Autodesk Inventor part; units mm, degrees
ref_plane "Work Plane1" through (0, 50, 0) normal (0, 1, 0) x (1, 0, 0)
ref_plane "YZ Plane" through (0, 0, 0) normal (1, 0, 0) x (0, 1, 0)
ref_plane "XZ Plane" through (0, 0, 0) normal (0, 1, 0) x (-1, 0, 0)
sketch "Sketch1" plane through (0, 0, 0) normal (0, 1, 0) x (-1, 0, 0)
  circle A0 centre (0, 0) radius 46
  dimension "d0" = 92
extrude "Extrusion1" add sketch "Sketch1" along normal blind 50
ref_plane "Work Plane1" through (0, 50, 0) normal (0, 1, 0) x (1, 0, 0)
sketch "Sketch2" plane through (0, 50, 0) normal (0, 1, 0) x (1, 0, 0)
  circle A0 centre (0, 0) radius 36
  dimension "d4" = 72
extrude "Extrusion2" cut sketch "Sketch2" against normal blind 40
sketch "Sketch3" plane through (0, 0, 0) normal (1, 0, 0) x (0, 1, 0)
  line L0 (50, -46) -> (0, -46)
  line L1 (0, -46) -> (0, 46)
  line L2 (0, 46) -> (50, 46)
  line L3 (50, 46) -> (50, 36)
  line L4 (50, 36) -> (10, 36)
  line L5 (10, 36) -> (10, -36)
  line L6 (10, -36) -> (50, -36)
  line L7 (50, -36) -> (50, -46)
  line L8 (0, 46) -> (50, 46)
  line L9 (10, 46) -> (5, 46)
  line L10 (5, 46) -> (5, 44)
  line L11 (5, 44) -> (10, 44)
  line L12 (10, 44) -> (10, 46)
  line L13 (20, 46) -> (15, 46)
  line L14 (15, 46) -> (15, 44)
  line L15 (15, 44) -> (20, 44)
  line L16 (20, 44) -> (20, 46)
  line L17 (-10, 0) -> (60, 0)
  point P0 (0, 0)
  point P1 (15, 46)
  dimension "d7" = 5
  dimension "d8" = 5
  dimension "d9" = 5
  dimension "d10" = 5
  dimension "d11" = 2
revolve "Revolution1" cut sketch "Sketch3" angle 360 about axis through (0, -10, 0) along (0, 1, 0) contours L2 L12 L11 L10 | L2 L16 L15 L14
sketch "Sketch4" plane through (0, 0, 0) normal (1, 0, 0) x (0, 1, 0)
  line L0 (10, -36) -> (50, -36)
  line L1 (50, -36) -> (50, -46)
  line L2 (50, -46) -> (20, -46)
  line L3 (20, -46) -> (20, -44)
  line L4 (20, -44) -> (15, -44)
  line L5 (15, -44) -> (15, -46)
  line L6 (15, -46) -> (10, -46)
  line L7 (10, -46) -> (10, -44)
  line L8 (10, -44) -> (5, -44)
  line L9 (5, -44) -> (5, -46)
  line L10 (5, -46) -> (0, -46)
  line L11 (0, -46) -> (0, 46)
  line L12 (0, 46) -> (5, 46)
  line L13 (5, 46) -> (5, 44)
  line L14 (5, 44) -> (10, 44)
  line L15 (10, 44) -> (10, 46)
  line L16 (10, 46) -> (15, 46)
  line L17 (15, 46) -> (15, 44)
  line L18 (15, 44) -> (20, 44)
  line L19 (20, 44) -> (20, 46)
  line L20 (20, 46) -> (50, 46)
  line L21 (50, 46) -> (50, 36)
  line L22 (50, 36) -> (10, 36)
  line L23 (10, 36) -> (10, -36)
  line L24 (10, -36) -> (50, -36)
  line L25 (50, -36) -> (50, -46)
  line L26 (50, 46) -> (50, 36)
  line L27 (50, 36) -> (10, 36)
  line L28 (10, 36) -> (10, -36)
  line L29 (20, -46) -> (20, 46)
  line L30 (50, -46) -> (50, 46)
  circle A0 centre (30, 0) radius 3.25
  line L31 (50, -46) -> (20, -46)
  line L32 (20, -46) -> (20, -44)
  line L33 (20, -44) -> (15, -44)
  line L34 (15, -44) -> (15, -46)
  line L35 (15, -46) -> (10, -46)
  line L36 (10, -46) -> (10, -44)
  line L37 (10, -44) -> (5, -44)
  line L38 (5, -44) -> (5, -46)
  line L39 (5, -46) -> (0, -46)
  line L40 (0, -46) -> (0, 46)
  line L41 (0, 46) -> (5, 46)
  line L42 (5, 46) -> (5, 44)
  line L43 (5, 44) -> (10, 44)
  line L44 (10, 44) -> (10, 46)
  line L45 (10, 46) -> (15, 46)
  line L46 (15, 46) -> (15, 44)
  line L47 (15, 44) -> (20, 44)
  line L48 (20, 44) -> (20, 46)
  line L49 (20, 46) -> (50, 46)
  point P0 (0, 0)
  dimension "d17" = 6.5
  dimension "d18" = 20
extrude "Extrusion3" cut sketch "Sketch4" along normal through all both and the other way through all contours A0
pattern_circular "Circular Pattern1" count 8 over 360 about axis through (0, 50, 0) along (0, -1, 0) of "Extrusion3"
properties part number "bulk head 94mm"
For this review, take the finished solid that the model builds, in its own axes (mm). A direction names the side the tool comes from. Round coordinates to 2 decimals unless told otherwise and drop trailing zeros. Loops run counter-clockwise (first coordinate to the right, second up) from the corner with the lowest first, then second, coordinate; pieces in that order, holes last. Notation, with made-up numbers: (1, 48.5) - (53, 48.5) arc R11 cw to (53, 67.5) - close; hole circle Ø11 at (-6, 11.25). An arc over 180 degrees is marked (long way). Put each result on its own line as item: value. Start each with the question number.
1. Consider section A-A on z = 0. State how many separate pieces and enclosed holes the cut face has, plus the area to 3 significant figures.
2. For probe 1 along Y at (x, z) = (0, 43); probe 2 along Z at (x, y) = (0, 23); probe 3 along X at (y, z) = (30, 42.5), list the stretches that pass through material, from the lowest coordinate up. Write a range as [from, to].
3. Mouldability with a two-part tool opening along Y and no side actions: class faces 4 (the cylindrical face through (29.58, 33.1, 28.2)), 5 (the flat face through (-1, 10, -1)), 6 (the cylindrical face through (5.99, 12.46, -45.61)) as +Y half, -Y half, draft (parallel to the pull), parting line (faces both ways), or undercut.
4. For faces 1 (the cylindrical face through (33.255, 30.28, 13.788)), 2 (the cylindrical face through (-42.954, 7.535, -9.538)), 3 (the cylindrical face through (0.98, 33.1, 40.86)), list the 3-axis set-ups (+Z, -Z, +X, -X, +Y, -Y) from which the entire face can be reached by the end or side of a thin tool; tool diameter is ignored.
5. Insertion check: P1, Ø1, axis at y = 16, z = -6.5, coming from the -X side; P2, Ø8, axis at x = -21.5, y = 14, coming from the +Z side; P3, Ø3, axis at x = -31, y = 7.5, coming from the -Z side. Each pin has a flat end and moves straight along its axis. Give the tip position at first contact, or say it passes through.
6. Consider section D-D on y = 45. State the section outline as (x, z) points, plus the area to 3 significant figures.
Result sheet:
1. separate pieces: 3
1. enclosed holes: 0
1. area: 1,550 mm^2
2. probe 1: [0, 26.75], [33.25, 50]
2. probe 2: [-46, -36], [36, 46]
2. probe 3: [-17.6, -3.25], [3.25, 17.6]
3. face 4: undercut
3. face 5: +Y half
3. face 6: draft
4. face 1: +Y
4. face 2: none
4. face 3: +Z, -Z
5. P1: x = -43.59
5. P2: z = 42.54
5. P3: z = -32.65
6. outline: circle Ø92 at (0, 0); hole circle Ø72 at (0, 0)
6. area: 2,580 mm^2
